Geometry: see drawing. Coordinates: mm, zero at the bounding-box minimum. Give positions to 0.01 mm unless a question says otherwise; leave off trailing zeros. Write each loop counter-clockwise with the first axis right and the second up, starting at its lowest first coordinate (ties: lowest second). Pieces come first, ordered by that corner, then holes.
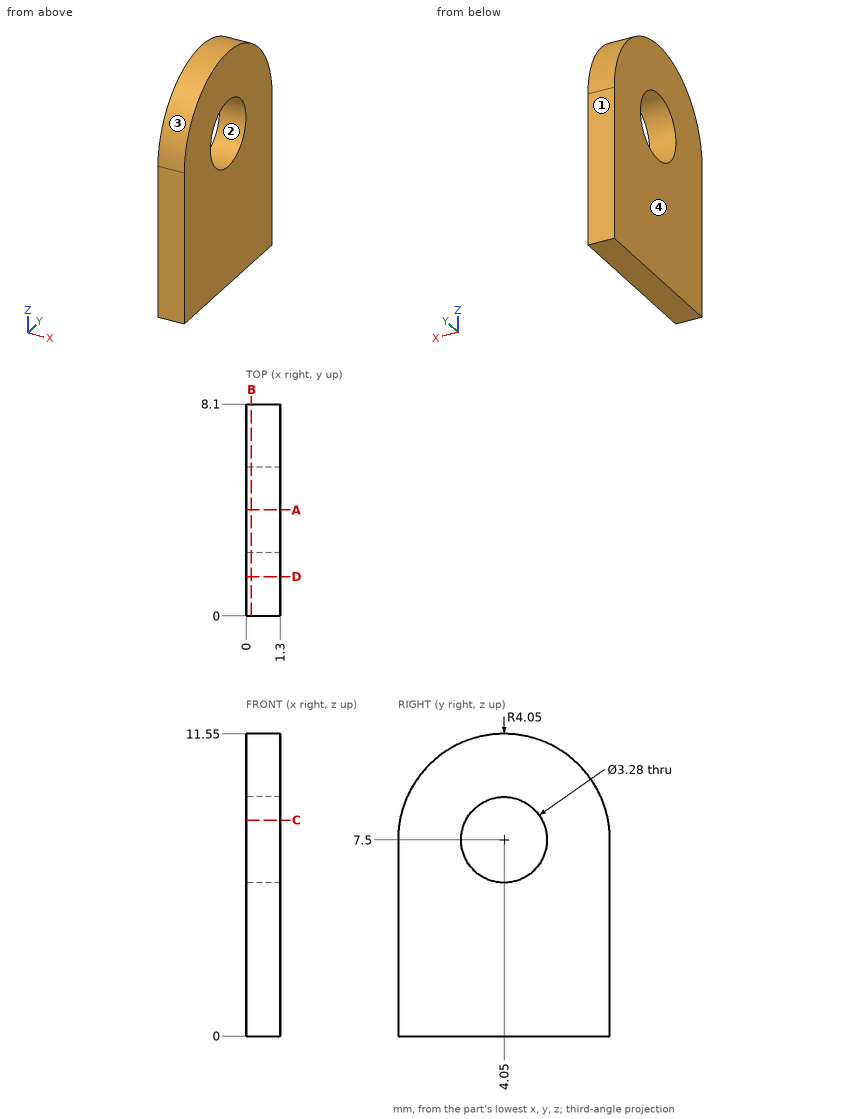
1. Pin query (flat end, axial travel): P1, Ø1, axis at y = 3, z = 2, coming from the -X side. Return the tip coordinate at first contact, or that it passes through.
2. Pull-direction query (Y, two-part tool) for the marked faces 1, 2, 3 and 4; classes: pulls with the +Y half, pulls with the -Y half, needs draft (parallel to the pull), parting line crosses it, or undercut.
3. Section query B-B (x = 0.2). Return loops of the section in (y, z), plus the area to 3 significant figures.
4. Section query A-A (y = 4.05). Return loops of the section in (x, z).
5. Section query C-C (z = 8.25). Return loops of the section in (x, y), plus the area to 3 significant figures.
6. Line query: probe 1 along Y at (x, z) = (0.95, 7.5); probe 2 along Z at (x, y) = (1, 4.05); probe 3 along Z at (x, y) = (0.15, 5.25). Output: solid intervals per line, ascending.
7. Section query D-D (y = 1.5). Return loops of the section in (x, z).
The answers:
1. P1: stops at x = 0
2. face 1: pulls with the +Y half
2. face 2: undercut
2. face 3: parting line crosses it
2. face 4: needs draft
3. outline: (0, 0) - (8.1, 0) - (8.1, 7.5) arc R4.05 ccw to (0, 7.5) - close; hole circle Ø3.28 at (4.05, 7.5)
3. area: 78.1 mm2
4. outline: (0, 0) - (1.3, 0) - (1.3, 5.86) - (0, 5.86) - close; (0, 9.14) - (1.3, 9.14) - (1.3, 11.55) - (0, 11.55) - close
5. outline: (0, 0.07) - (1.3, 0.07) - (1.3, 2.59) - (0, 2.59) - close; (0, 5.51) - (1.3, 5.51) - (1.3, 8.03) - (0, 8.03) - close
5. area: 6.56 mm2
6. probe 1: y = 0 to 2.41, 5.69 to 8.1
6. probe 2: z = 0 to 5.86, 9.14 to 11.55
6. probe 3: z = 0 to 6.38, 8.62 to 11.37
7. outline: (0, 0) - (1.3, 0) - (1.3, 10.65) - (0, 10.65) - close
